Can you work these out from the drawing? Everything is in mm from the part's minimum corner. A direction names the side the tool comes from. Give positions to 0.01 mm unless a question says otherwise; leave off trailing zeros. Loops run counter-clockwise (first coordinate to the right, second up) from the corner with the lowest first, then second, coordinate; pieces in that order, holes last. Notation, with made-up numbers: (58, 78) -> (68, 78) arc R9 cw to (68, 89) -> close; hole circle Ø11 at (-25, 20). An arc over 180 degrees is marked (long way). Return JSON: item names as keys, results as strings. Group by question number.
Q1. I need wall thicknesses on line 1 along X through (y, z) = (5.5, 7.5) (1 decimal); line 2 along X through (y, z) = (4.75, 5) (1 decimal); line 3 along X through (y, z) = (0.5, 0.75) (1 decimal). Which ranges of each line are inside material? Lowest first, please. Write a range as [from, to].
Q2. Suppose I cut it at A-A, the plane y = 4.75. Please give me the cut outline in (x, z) (1 decimal).
Q3. Suppose I cut it at D-D, the plane x = 72. Please give me the cut outline in (y, z), and give its area (3 significant figures).
Q4. Thinking about a two-plate mould opening in X: for the marked faces 3, 4 and 5, which applies, pulls with the +X half, pulls with the -X half, needs draft (parallel to the pull), parting line crosses it, or undercut?
Q5. Suppose I cut it at C-C, the plane x = 35. Please give me the cut outline in (y, z).
Q6. Suppose I cut it at B-B, the plane z = 4.75. Count the separate pieces of the cut face and the enclosed holes in it.
Q7. Which directions (+Z, -Z, +X, -X, +Y, -Y) give clear straight access to the entire face, cutting with the end or side of a thin tool? Please do the marked faces 1 and 2.
Q8. Will these pins go through, and if not, where does the flat tip stop? pin 1 (4 mm diameter, centred on x = 76.5, z = 2.5, fed in from -Y); pin 2 (2 mm diameter, centred on x = 19.5, z = 1.5, fed in from -Y); pin 3 (2.5 mm diameter, centred on x = 4, z = 3.5, fed in from +Y).
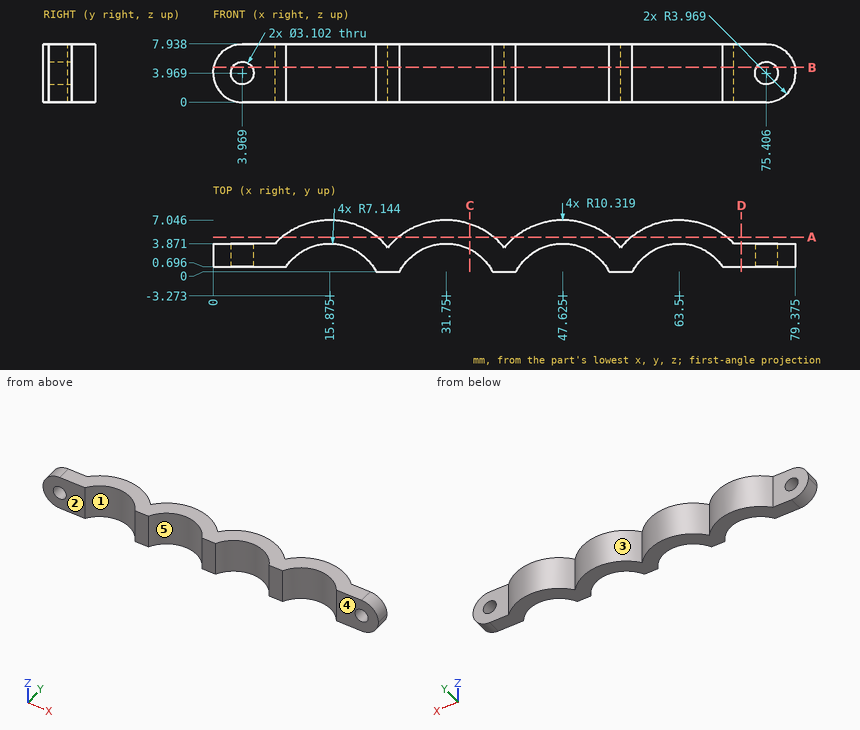
Ans:
{
 "1": {"line 1": "x = [10.4, 21.3], [26.3, 37.2], [42.2, 53.1], [58.1, 68.9]", "line 2": "x = [9.4, 22.4], [25.3, 38.2], [41.1, 54.1], [57, 70]", "line 3": "x = [21.9, 25.7], [37.8, 41.6], [53.7, 57.4]"},
 "2": {"outline": "(9.4, 0) -> (22.4, 0) -> (22.4, 7.9) -> (9.4, 7.9) -> close; (25.3, 0) -> (38.2, 0) -> (38.2, 7.9) -> (25.3, 7.9) -> close; (41.1, 0) -> (54.1, 0) -> (54.1, 7.9) -> (41.1, 7.9) -> close; (57, 0) -> (70, 0) -> (70, 7.9) -> (57, 7.9) -> close"},
 "3": {"outline": "(0.7, 0) -> (3.87, 0) -> (3.87, 7.94) -> (0.7, 7.94) -> close", "area": "25.2 mm^2"},
 "4": {"face 3": "undercut", "face 4": "needs draft", "face 5": "undercut"},
 "5": {"outline": "(3.09, 0) -> (6.52, 0) -> (6.52, 7.94) -> (3.09, 7.94) -> close"},
 "6": {"separate pieces": "3", "enclosed holes": "0"},
 "7": {"face 1": "+Z, -Z, -Y", "face 2": "+Z, -Z, -X, -Y"},
 "8": {"pin 1": "stops at y = 0.7", "pin 2": "stops at y = 2.17", "pin 3": "stops at y = 3.87"}
}
